CAD build for the part. Positions are in the model's coordinates, mm. Round coordinates to 2 decimals unless told otherwise and drop trailing zeros. Order: outer loops, then holes, each group sorted by start corner. A loop starts at its lowest first (then second) coordinate and runs counter-clockwise, first axis right, second up. Notation, with made-up numbers: (50.5, 66) -> (79.5, 66) arc R21 cw to (79.5, 81) -> close; hole circle Ø9 at (-11, 2.25). An arc over 180 degrees is marked (long way). Return JSON: item names as keys, results as strings. Group by question number.
Q1. Mould opens along X. For faces 1 (the cylindrical face through (1.84, 54.97, 0.49)), 2 (the cylindrical face through (-4.686, 35.694, 0.493)), 3 (the flat face through (-1, 40, 0)) say: +X half, -X half, draft (parallel to the pull), parting line (faces both ways), or undercut.
Q2. Cut at D-D (y = -22.5). Write the cut outline in (x, z).
Q3. Cut at B-B (x = 19.5). Write the cut outline in (y, z).
Q4. Probe line 1 along Y through (x, z) = (0, 0.2); line 2 along X through (y, z) = (-7, 0.75); line 3 along Y through (x, z) = (12.5, 0.15). List the from-to ranges inside material, lowest first.
Q5. Cut at A-A (y = 0). Write the cut outline in (x, z), then the cut area to 3 significant figures.
Q6. Cut at C-C (z = 0.4). Write the cut outline in (x, y), then the cut area to 3 significant figures.
from build123d import *

# Parameters (mm, degrees)
SCHIZZO1_R                   = 55
SCHIZZO1_R_2                 = 36
ESTRUSIONE_ESTRUSIONE1_DEPTH = 1
SCHIZZO2_R                   = 4.5
TAGLIO_ESTRUSIONE1_DEPTH     = 78.788173908
SCHIZZO4_OUTSIDE_W           = 143.114
SCHIZZO4_OUTSIDE_H           = 143.114
TAGLIO_ESTRUSIONE2_DEPTH     = 78.788173908


with BuildPart() as part:
    # Schizzo1 → Estrusione-Estrusione1 (new body)
    with BuildSketch(Plane.XY):
        Circle(SCHIZZO1_R)
        Circle(SCHIZZO1_R_2, mode=Mode.SUBTRACT)
    extrude(amount=ESTRUSIONE_ESTRUSIONE1_DEPTH)

    # Schizzo2 → Taglio-Estrusione1 (cut, through all)
    with BuildSketch(Plane.XY.offset(1)):
        with Locations((0, 45)):
            Circle(SCHIZZO2_R)
        with Locations((38.97114317, -22.5)):
            Circle(SCHIZZO2_R)
        with Locations((-38.97114317, -22.5)):
            Circle(SCHIZZO2_R)
    extrude(amount=-TAGLIO_ESTRUSIONE1_DEPTH, mode=Mode.SUBTRACT)

    # Schizzo4 outside → Taglio-Estrusione2 (cut, through all)
    with BuildSketch(Plane.XY):
        Rectangle(SCHIZZO4_OUTSIDE_W, SCHIZZO4_OUTSIDE_H)
        with BuildLine():
            Line((37.749172176, -40), (-37.749172176, -40))
            ThreePointArc((-37.749172176, -40), (0, 55), (37.749172176, -40))
        make_face(mode=Mode.SUBTRACT)
    extrude(amount=TAGLIO_ESTRUSIONE2_DEPTH, mode=Mode.SUBTRACT)


solid = part.part
Solution:
{
 "1": {"face 1": "parting line", "face 2": "undercut", "face 3": "draft"},
 "2": {"outline": "(-50.19, 0) -> (-43.47, 0) -> (-43.47, 1) -> (-50.19, 1) -> close; (-34.47, 0) -> (-28.1, 0) -> (-28.1, 1) -> (-34.47, 1) -> close; (28.1, 0) -> (34.47, 0) -> (34.47, 1) -> (28.1, 1) -> close; (43.47, 0) -> (50.19, 0) -> (50.19, 1) -> (43.47, 1) -> close"},
 "3": {"outline": "(-40, 0) -> (-30.26, 0) -> (-30.26, 1) -> (-40, 1) -> close; (30.26, 0) -> (51.43, 0) -> (51.43, 1) -> (30.26, 1) -> close"},
 "4": {"line 1": "y = -40 to -36, 36 to 40.5, 49.5 to 55", "line 2": "x = -54.55 to -35.31, 35.31 to 54.55", "line 3": "y = -40 to -33.76, 33.76 to 53.56"},
 "5": {"outline": "(-55, 0) -> (-36, 0) -> (-36, 1) -> (-55, 1) -> close; (36, 0) -> (55, 0) -> (55, 1) -> (36, 1) -> close", "area": "38.0 mm²"},
 "6": {"outline": "(-37.75, -40) -> (37.75, -40) arc R55 ccw (long way) to start; hole circle Ø9 at (-38.97, -22.5); hole circle Ø72 at (0, 0); hole circle Ø9 at (0, 45); hole circle Ø9 at (38.97, -22.5)", "area": "4,460 mm²"}
}
